Input: part model. Units: mm. Frame: model coordinates. A direction names the side the tool comes from. Coordinates: 2 decimals unless noted, no trailing zeros. Write each loop counter-clockwise with the first axis right and the second up, starting at its lowest first coordinate (ties: lowest second). Pieces come first, ordered by that corner, then holes. Notation, with made-up numbers: M 38,12.5 L 94,12.5 A22 cw 94,19.5 Z; hole C 9.25,7 d8. An arc over 180 degrees is marked long. Answer as a JSON object with one key per item and string values. Group by question number.
from build123d import *

# Parameters (mm, degrees)
SKETCH1_W           = 4
SKETCH1_H           = 2
BOSS_EXTRUDE1_DEPTH = 4


with BuildPart() as part:
    # Sketch1 → Boss-Extrude1 (new body)
    with BuildSketch(Plane.XY):
        with BuildLine():
            Line((14.475572066, 6), (15.475572066, 7.732050808))
            Line((15.475572066, 7.732050808), (17.939673681, 6.309401077))
            Line((17.939673681, 6.309401077), (17.939673681, 13.142551265))
            ThreePointArc((17.939673681, 13.142551265), (16.768100806, 15.97097839), (13.939673681, 17.142551265))
            Line((13.939673681, 17.142551265), (10.920326319, 17.142551265))
            ThreePointArc((10.920326319, 17.142551265), (6.2, 20.055557209), (1.479673681, 17.142551265))
            Line((1.479673681, 17.142551265), (-1.520326319, 17.142551265))
            Line((-1.520326319, 17.142551265), (-1.520326319, 2.09107808))
            Line((-1.520326319, 2.09107808), (16.939673681, 2.09107808))
            Line((16.939673681, 2.09107808), (16.939673681, 4.577350269))
            Line((16.939673681, 4.577350269), (14.475572066, 6))
        make_face()
        with Locations((5.5, 9.99107808)):
            Rectangle(SKETCH1_W, SKETCH1_H, mode=Mode.SUBTRACT)
        with Locations((13.5, 9.99107808)):
            Rectangle(SKETCH1_W, SKETCH1_H, mode=Mode.SUBTRACT)
        Polygon((2.95, 14.774571729), (4.575, 11.959989167), (7.825, 11.959989167), (9.45, 14.774571729), (7.825, 17.589154291), (4.575, 17.589154291), align=None, mode=Mode.SUBTRACT)
    extrude(amount=BOSS_EXTRUDE1_DEPTH)


solid = part.part
Q1. Section D-D, the plane x = 4. Return the cut outline in (y, z).
Q2. Line query: line 1 (X direction, y = 10.75, z = 2.2); line 2 (Y direction, x = 5.5, z = 3.5); line 3 (Y direction, x = 14, z = 1.6). Output: solid intervals per line, ascending. Write a range as from..to.
Q3. Pin query (flat end, axial travel): pin 1 Ø2 at (x, z) = (4.5, 1) entering from +Y; pin 2 Ø2 at (y, z) = (3, 2.5) entering from +X; pin 3 Ø1.2 at (x, z) = (14, 1) entering from +Y. Return the tip coordinate at first contact, or that it passes through.
Q4. Draft query along Y for faces 4 (the flat face through (8, 2.091, 2)), 5 (the flat face through (7.5, 10, 2)), 6 (the flat face through (17.94, 10, 2)). Return one class per face: released by +Y, released by -Y, zero draft, split by the parting line, or undercut.
Q5. Section A-A, the plane y = 10.5. Return the cut outline in (x, z).
Q6. Section B-B, the plane z = 2.6. Return the cut outline in (x, y) (3 decimals).
Q7. Section C-C, the plane x = 8.5. Return the cut outline in (y, z), and give its area (3 significant figures).
Q8. Access query for faces 1 (the flat face through (12, 17.143, 2)), 2 (the flat face through (15.72, 5.28, 1.97)), 3 (the flat face through (16.69, 7.03, 1.97)). Directions: +Z, -Z, +X, -X, +Y, -Y. A direction counts if a zero-diameter tool reaches every point of the face in a straight line with its end or side. Return the directions, or none.
Filled in:
{
 "1": {"outline": "M 2.09,0 L 8.99,0 L 8.99,4 L 2.09,4 Z; M 10.99,0 L 12.96,0 L 12.96,4 L 10.99,4 Z; M 16.59,0 L 19.58,0 L 19.58,4 L 16.59,4 Z"},
 "2": {"line 1": "-1.52..3.5, 7.5..11.5, 15.5..17.94", "line 2": "2.09..8.99, 10.99..11.96, 17.59..20.01", "line 3": "2.09..8.99, 10.99..17.14"},
 "3": {"pin 1": "y = 20.01", "pin 2": "x = 16.94", "pin 3": "y = 17.14"},
 "4": {"face 4": "released by -Y", "face 5": "undercut", "face 6": "zero draft"},
 "5": {"outline": "M -1.52,0 L 3.5,0 L 3.5,4 L -1.52,4 Z; M 7.5,0 L 11.5,0 L 11.5,4 L 7.5,4 Z; M 15.5,0 L 17.94,0 L 17.94,4 L 15.5,4 Z"},
 "6": {"outline": "M -1.52,2.091 L 16.94,2.091 L 16.94,4.577 L 14.476,6 L 15.476,7.732 L 17.94,6.309 L 17.94,13.143 A4 ccw 13.94,17.143 L 10.92,17.143 A5.281 ccw 1.48,17.143 L -1.52,17.143 Z; hole M 2.95,14.775 L 4.575,11.96 L 7.825,11.96 L 9.45,14.775 L 7.825,17.589 L 4.575,17.589 Z; hole M 3.5,8.991 L 7.5,8.991 L 7.5,10.991 L 3.5,10.991 Z; hole M 11.5,8.991 L 15.5,8.991 L 15.5,10.991 L 11.5,10.991 Z"},
 "7": {"outline": "M 2.09,0 L 13.13,0 L 13.13,4 L 2.09,4 Z; M 16.42,0 L 19.53,0 L 19.53,4 L 16.42,4 Z", "area": "56.6 mm^2"},
 "8": {"face 1": "+Z, -Z, +X, +Y", "face 2": "+Z, -Z, +X", "face 3": "+Z, -Z"}
}
